```python
from build123d import *

# Parameters (mm, degrees)
SKETCH_1_W          = 80
SKETCH_1_H          = 38
SKETCH_1_W_2        = 45.5
SKETCH_1_H_2        = 27
SKETCH_1_W_3        = 12
SKETCH_1_H_3        = 19.5
EXTRUDE_1_DEPTH     = 3
EXTRUDE_2_DEPTH     = 4
EXTRUDE_START       = -49.5
EXTRUDE_3_DEPTH     = 4
EXTRUDE_START_2     = -76
EXTRUDE_4_DEPTH     = 4
SKETCH_6_W          = 80
SKETCH_6_H          = 37
EXTRUDE_5_DEPTH     = 3
SKETCH_7_R          = 1.6
CUT_EXTRUDE_1_DEPTH = 80.501880139


with BuildPart() as part:
    # 草图1 → 凸台-拉伸1 (new body)
    with BuildSketch(Plane.XY):
        Rectangle(SKETCH_1_W, SKETCH_1_H)
        with Locations((-13.25, 0)):
            Rectangle(SKETCH_1_W_2, SKETCH_1_H_2, mode=Mode.SUBTRACT)
        with Locations((26, -0.838945713)):
            Rectangle(SKETCH_1_W_3, SKETCH_1_H_3, mode=Mode.SUBTRACT)
    extrude(amount=EXTRUDE_1_DEPTH)

    # 草图3 → 凸台-拉伸2 (add)
    with BuildSketch(Plane.ZY.offset(40)):
        with BuildLine():
            Line((3, 19), (3, 24))
            Line((3, 24), (-2.773502692, 34))
            Line((-2.773502692, 34), (-34.816442632, 52.5))
            ThreePointArc((-34.816442632, 52.5), (-38.437762975, 52.023244132), (-38.914518843, 48.401923789))
            Line((-38.914518843, 48.401923789), (0, -19))
            Line((0, -19), (0, 19))
            Line((0, 19), (3, 19))
        make_face()
    extrude(amount=-EXTRUDE_2_DEPTH)

    # 草图4 → 凸台-拉伸3 (add)
    with BuildSketch(Plane.ZY.offset(40).offset(EXTRUDE_START)):
        with BuildLine():
            Line((-38.914518843, 48.401923789), (0, -19))
            Line((0, -19), (3, -19))
            Line((3, -19), (3, 24))
            Line((3, 24), (-2.773502692, 34))
            Line((-2.773502692, 34), (-34.816442632, 52.5))
            ThreePointArc((-34.816442632, 52.5), (-38.437762975, 52.023244132), (-38.914518843, 48.401923789))
        make_face()
    extrude(amount=-EXTRUDE_3_DEPTH)

    # 草图5 → 凸台-拉伸4 (add)
    with BuildSketch(Plane.ZY.offset(40).offset(EXTRUDE_START_2)):
        with BuildLine():
            Line((-38.914518843, 48.401923789), (0, -19))
            Line((0, -19), (3, -19))
            Line((3, -19), (3, 24))
            Line((3, 24), (-2.773502692, 34))
            Line((-2.773502692, 34), (-34.816442632, 52.5))
            ThreePointArc((-34.816442632, 52.5), (-38.437762975, 52.023244132), (-38.914518843, 48.401923789))
        make_face()
    extrude(amount=-EXTRUDE_4_DEPTH)

    # 草图6 → 凸台-拉伸5 (add)
    with BuildSketch(Plane(origin=(0, 24.299038106, 14.029056191), x_dir=(1, 0, 0), z_dir=(0, 0.86602540378444, 0.4999999999999976))):
        with Locations((0, 37.901923789)):
            Rectangle(SKETCH_6_W, SKETCH_6_H)
    extrude(amount=-EXTRUDE_5_DEPTH)

    # 草图7 → 切除-拉伸1 (cut, through all)
    with BuildSketch(Plane(origin=(0, 24.299038106, 14.029056191), x_dir=(1, 0, 0), z_dir=(0, 0.86602540378444, 0.4999999999999975))):
        with Locations(Location((-24.625, 47.901923789, 0), (0, 0, 270))):
            Circle(SKETCH_7_R)
        with Locations(Location((-1.875, 47.901923789, 0), (0, 0, 270))):
            Circle(SKETCH_7_R)
        with Locations(Location((-1.875, 27.901923789, 0), (0, 0, 270))):
            Circle(SKETCH_7_R)
        with Locations(Location((-24.625, 27.901923789, 0), (0, 0, 270))):
            Circle(SKETCH_7_R)
        with Locations(Location((24.75, 47.901923789, 0), (0, 0, 270))):
            Circle(SKETCH_7_R)
        with Locations(Location((24.75, 27.901923789, 0), (0, 0, 270))):
            Circle(SKETCH_7_R)
        with Locations(Location((-27, 33.401923789, 0), (0, 0, 270))):
            Circle(SKETCH_7_R)
        with Locations(Location((27, 33.401923789, 0), (0, 0, 270))):
            Circle(SKETCH_7_R)
        with Locations(Location((-27, 43.401923789, 0), (0, 0, 270))):
            Circle(SKETCH_7_R)
        with Locations(Location((27, 43.401923789, 0), (0, 0, 270))):
            Circle(SKETCH_7_R)
    extrude(amount=-CUT_EXTRUDE_1_DEPTH, mode=Mode.SUBTRACT)


solid = part.part
```
Check sheet for the modelled part. Datum: model origin and axes. Units: mm. A direction names the side the tool comes from. Round coordinates to 2 decimals unless told otherwise and drop trailing zeros. Loops run counter-clockwise (first coordinate to the right, second up) from the corner with the lowest first, then second, coordinate; pieces in that order, holes last. Notation, with made-up numbers: (51, -28) -> (62, -28) arc R22 ccw to (62, -21) -> close; hole circle Ø1 at (53.5, 50.25). An arc over 180 degrees is marked (long way). Write item = value, one per line. Start each with the question number.
1) Release check for a two-part mould opening along Z. For faces 1 (the cylindrical face through (24.82, 47.77, -29.58)), 2 (the cylindrical face through (11.47, 52.06, -38.4)), 3 (the flat face through (-14, 19, 1)) record: released by +Z, released by -Z, zero draft, split by the parting line, or undercut.
2) Sectioned sample at B-B, the plane y = -3. Record the cut outline in (x, z).
3) Gauge pin test, flat ends, axial feed: pin 1 Ø10 at (x, y) = (23, 45) entering from -Z; pin 2 Ø2 at (x, y) = (29, -11) entering from -Z; pin 3 Ø3.5 at (x, z) = (-18, 2) entering from +Y; pin 4 Ø21 at (y, z) = (7, -20) entering from -X. Record the tip position at first contact, or that the pin passes through.
4) Thickness scan on probe 1 along X at (y, z) = (19.5, -15.5); probe 2 along Y at (x, z) = (-32, 1); probe 3 along Z at (x, y) = (35.5, 8). Record the ranges inside material, lowest first.
5) Sectioned sample at D-D, the plane z = -7.5. Record the cut outline in (x, y), plus the area to 3 significant figures.
6) Sectioned sample at A-A, the plane x = -17.5. Record the cut outline in (y, z), plus the area to 3 significant figures.
7) Sectioned sample at C-C, the plane z = -21. Record the cut outline in (x, y).
8) Set-up check for faces 4 (the cylindrical face through (37.97, 52.06, -38.4)), 5 (the cylindrical face through (-23.04, 47.07, -28.38)), 6 (the flat face through (26, 8.911, 1)), 7 (the flat face through (-13.568, 32.719, -3.513)), 8 (the flat face through (19.6, 0.3, 0)): record each of +Z, -Z, +X, -X, +Y, -Y from which the full face is reachable in a straight line by a thin tool's end or side.
Results are:
q1.face_1 = undercut
q1.face_2 = split by the parting line
q1.face_3 = zero draft
q2.outline = (-40, -9.24) -> (-36, -9.24) -> (-36, 3) -> (-40, 3) -> close; (9.5, -9.24) -> (13.5, -9.24) -> (13.5, 0) -> (20, 0) -> (20, 3) -> (9.5, 3) -> close; (32, 0) -> (36, 0) -> (36, -9.24) -> (40, -9.24) -> (40, 3) -> (32, 3) -> close
q3.pin_1 = -36.32
q3.pin_2 = 0
q3.pin_3 = 19
q3.pin_4 = -40
q4.probe_1 = -40 to -36, 9.5 to 13.5, 36 to 40
q4.probe_2 = -19 to -13.5, 13.5 to 19
q4.probe_3 = 0 to 3
q5.outline = (-40, -6.01) -> (-36, -6.01) -> (-36, 33.26) -> (9.5, 33.26) -> (9.5, -6.01) -> (13.5, -6.01) -> (13.5, 33.26) -> (36, 33.26) -> (36, -6.01) -> (40, -6.01) -> (40, 36.73) -> (-40, 36.73) -> close
q5.area = 748 mm^2
q6.outline = (-19, 0) -> (-13.5, 0) -> (-13.5, 3) -> (-19, 3) -> close; (13.5, 0) -> (19, 0) -> (19, 3) -> (13.5, 3) -> close; (31.4, -4.27) -> (49.9, -36.32) -> (52.5, -34.82) -> (34, -2.77) -> close
q6.area = 144 mm^2
q7.outline = (-40, 17.37) -> (-36, 17.37) -> (-36, 41.06) -> (9.5, 41.06) -> (9.5, 17.37) -> (13.5, 17.37) -> (13.5, 41.06) -> (36, 41.06) -> (36, 17.37) -> (40, 17.37) -> (40, 44.52) -> (-40, 44.52) -> close
q8.face_4 = +X, -X
q8.face_5 = none
q8.face_6 = +Z, -Z
q8.face_7 = +Z, -Y
q8.face_8 = -Z, +Y, -Y
